Read the model definition and answer for the solid it produces. Units are mm, in the model's axes. Coordinates: 2 decimals unless noted, no trailing zeros. Write each loop counter-clockwise with the first axis right and the second up, starting at its lowest first coordinate (ties: lowest second). Pieces come first, ordered by that corner, then holes. Notation, with made-up numbers: (61.25, -34.5) -> (104.25, -34.5) arc R12 ccw to (104.25, -24.5) -> close; hole circle Ø3 at (23, -0.5). An arc over 180 degrees is marked (long way). Use CSV: the item, a comma, the result in double quotes.
Autodesk Inventor part; units mm, degrees
ref_plane "YZ Plane" through (0, 0, 0) normal (1, 0, 0) x (0, 1, 0)
ref_plane "XZ Plane" through (0, 0, 0) normal (0, 1, 0) x (-1, 0, 0)
ref_plane "XY Plane" through (0, 0, 0) normal (0, 0, 1) x (1, 0, 0)
sketch "Sketch1" plane through (0, 0, 0) normal (0, 0, 1) x (1, 0, 0)
  circle A0 centre (0, 0) radius 300
  dimension "d0" = 600
extrude "Plate1" add sketch "Sketch1" against normal blind 4
sketch "Sketch2" plane through (0, 0, 0) normal (0, 0, 1) x (1, 0, 0)
  circle A0 centre (0, 0) radius 275 construction
  circle A1 centre (0, 275) radius 8.5
  dimension "d2" = 550
  dimension "d3" = 17
extrude "Extrusion1" cut sketch "Sketch2" against normal through all
pattern_circular "Circular Pattern1" count 24 over 360 about axis through (0, 0, -10) along (0, 0, 1) of "Extrusion1"
equation "\"d1\" = Thickness"
equation "\"BendReliefWidth\" = Thickness"
equation "\"BendReliefDepth\" = 0.5 * Thickness"
equation "\"CornerReliefSize\" = 4 * Thickness"
equation "\"MinimumRemnant\" = 2 * Thickness"
equation "\"TransitionRadius\" = BendRadius"
equation "\"JacobiRadiusSize\" = BendRadius"
equation "\"GapSize\" = Thickness"
properties part number "MSC 404 flange cover 500" material "Stainless Steel"
1. A cutting plane is placed at C-C (z = -2.15). Give the number of separate pieces and of enclosed holes in the cut face, and give its area (3 significant figures).
Solutions:
separate pieces,"1"
enclosed holes,"24"
area,"277,000 mm^2"
2. A cutting plane is placed at B-B (x = 0). Give the vertices of the cut face in (y, z).
Solutions:
outline,"(-300, -4) -> (-283.5, -4) -> (-283.5, 0) -> (-300, 0) -> close; (-266.5, -4) -> (266.5, -4) -> (266.5, 0) -> (-266.5, 0) -> close; (283.5, -4) -> (300, -4) -> (300, 0) -> (283.5, 0) -> close"
3. A cutting plane is placed at A-A (y = -137.5). Give the vertices of the cut face in (x, z).
Solutions:
outline,"(-266.63, -4) -> (-246.66, -4) -> (-246.66, 0) -> (-266.63, 0) -> close; (-229.66, -4) -> (229.66, -4) -> (229.66, 0) -> (-229.66, 0) -> close; (246.66, -4) -> (266.63, -4) -> (266.63, 0) -> (246.66, 0) -> close"
4. For a pull along Y with two mould halves and no side action, classify faces 1 (the cylindrical face through (231.41, -142.67, -1.97)), 2 (the flat face through (-4, 4, -4)) as pulls with the +Y half, pulls with the -Y half, needs draft (parallel to the pull), parting line crosses it, or undercut.
Solutions:
face 1,"undercut"
face 2,"needs draft"
5. A cutting plane is placed at D-D (y = 158.5). Give the vertices of the cut face in (x, z).
Solutions:
outline,"(-254.71, -4) -> (254.71, -4) -> (254.71, 0) -> (-254.71, 0) -> close"
6. Find the intervals of material crossed by line 1 along Y through (x, z) = (-71, -2); line 2 along X through (y, z) = (-68, -1.3); line 3 along X through (y, z) = (269, -1.95), in increasing order.
Solutions:
line 1,"y = -291.48 to -274.13, -257.13 to 257.13, 274.13 to 291.48"
line 2,"x = -292.19 to -273.51, -257.74 to 257.74, 273.51 to 292.19"
line 3,"x = -132.81 to -78.98, -63.37 to -6.02, 6.02 to 63.37, 78.98 to 132.81"
